CAD build for the part. Positions are in the model's coordinates, mm. Face numbers are marked on the shaded views. A direction names the side the tool comes from. Round coordinates to 2 decimals unless told otherwise and drop trailing zeros. Loops run counter-clockwise (first coordinate to the right, second up) from the corner with the lowest first, then second, coordinate; pieces in that order, holes last. Notation, with made-up numbers: M 73.25,-35 L 85.25,-35 A21 cw 85.25,-25 Z; hole C -8,87.25 d4. An arc over 180 degrees is marked long. Use one line per item in the form item = value.
from build123d import *

# Parameters (mm, degrees)
ESQUISSE1_W      = 80
ESQUISSE1_H      = 80
EXTRUSION1_DEPTH = 80
COQUE1_T         = -5


with BuildPart() as part:
    # Esquisse1 → Extrusion1 (new body)
    with BuildSketch(Plane(origin=(0, 0, 0), x_dir=(1, 0, 0), z_dir=(0, 1, 0))):
        with Locations((40, 40)):
            Rectangle(ESQUISSE1_W, ESQUISSE1_H)
    extrude(amount=EXTRUSION1_DEPTH)

    # Coque1
    coque1_openings = [part.faces().sort_by_distance(p)[0] for p in [
        (40, 0, -40),
    ]]
    offset(amount=COQUE1_T, openings=coque1_openings, kind=Kind.INTERSECTION)


solid = part.part
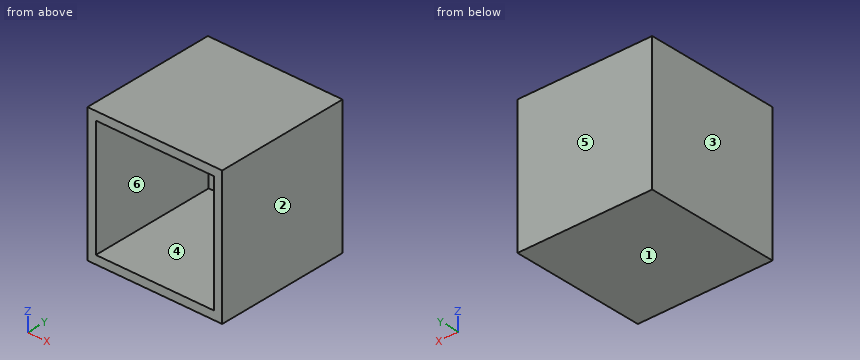
1. Cut at C-C on x = 29. Write the cut outline in (y, z), and give its area (3 significant figures).
Completed:
outline = M 0,-80 L 80,-80 L 80,0 L 0,0 L 0,-5 L 75,-5 L 75,-75 L 0,-75 Z
area = 1,150 mm2
2. Probe line 1 along Z through (x, y) = (70.5, 35.5); line 2 along X through (y, z) = (36, -19); line 3 along Y through (x, z) = (17.5, -9.5). List the from-to ranges inside material, lowest first. Write a range as from..to.
Completed:
line_1 = -80..-75, -5..0
line_2 = 0..5, 75..80
line_3 = 75..80
3. Drop a flat-ended pin along its axis: P1, Ø8, axis at x = 47, z = -61, coming from the -Y side. Give the stop position or say it passes through.
Completed:
P1 = 75
4. Tool access for the marked faces 5 and 6: list every direction of +Z, -Z, +X, -X, +Y, -Y with a clear straight run to the whole face (end or side of a thin tool).
Completed:
face_5 = +Z, -Z, +X, -X, +Y
face_6 = -Y
5. Cut at B-B on z = -13. Write the cut outline in (x, y), and give its area (3 significant figures).
Completed:
outline = M 0,0 L 5,0 L 5,75 L 75,75 L 75,0 L 80,0 L 80,80 L 0,80 Z
area = 1,150 mm2
6. Pull direction X, two halves, no side cores. Call the marked faces 1, 2, 3 and 4: +X half, -X half, draft (parallel to the pull), parting line (faces both ways), or undercut.
Completed:
face_1 = draft
face_2 = +X half
face_3 = -X half
face_4 = undercut
7. Cut at A-A on y = 61.5. Write the cut outline in (x, z).
Completed:
outline = M 0,-80 L 80,-80 L 80,0 L 0,0 Z; hole M 5,-75 L 75,-75 L 75,-5 L 5,-5 Z
